Design review of the part built by this model. Coordinates are the model's own, in mm. A direction names the side the tool comes from. Coordinates: 2 decimals unless noted, no trailing zeros. Write each loop counter-clockwise with the first axis right and the second up, starting at its lowest first coordinate (ties: lowest second). Pieces come first, ordered by that corner, then holes.
Q1. Clearance check with flat-ended pins moving along their axes: pin 1 Ø1.5 at (x, y) = (-10, 11.5) entering from -Z; pin 2 Ø11 at (x, z) = (-7.5, 50) entering from +Y; pin 3 Ø8 at (x, z) = (-38, -37) entering from +Y (3 decimals); pin 4 Ø2 at (x, z) = (-34.925, 34.925) entering from -Y. State where each tip first meets the part, or that it passes through.
Q2. Add section B-B, the plane y = 13. Give the boundary of the cut face in (x, z) (3 decimals), plus the area to 3 significant figures.
Q3. Machinability: for faces 1 (the face through (-41, 6.35, -41)), 2 (the face through (47.625, 3, -32)), 3 (the face through (35.274, 4.994, -42.855)), which of the approach directions +Z, -Z, +X, -X, +Y, -Y give a long, thin tool a straight path to every point of the face, cutting with its end or side? Answer none if there is none.
Q4. To check wall thickness, follow probe 1 along Z at (x, y) = (-25, 6.75); probe 2 along X at (y, z) = (7.75, 26); probe 3 along Y at (x, z) = (-9, 43). State the ranges of each line that lie inside material, in increasing order.
from build123d import *

# Parameters (mm, degrees)
SKETCH1_W               = 95.25
SKETCH1_H               = 95.25
SKETCH1_R               = 37.465
BOSS_EXTRUDE1_DEPTH     = 6.35
SKETCH2_R               = 1.75
CUT_EXTRUDE1_DEPTH      = 68.650600515
CIRPATTERN1_COUNT       = 4
FILLET1_R               = 12.7
FILLET2_R               = 3.175
SKETCH5_R               = 55.5625
SKETCH5_R_2             = 44.45
SKETCH5_R_3             = 1.75
BOSS_EXTRUDE2_DEPTH     = 6.35
BOSS_EXTRUDE4_START     = 1.5875
SKETCH8_R               = 55.5625
SKETCH8_R_2             = 52.3875
BOSS_EXTRUDE4_DEPTH     = 1.5875
CUT_EXTRUDE3_DEPTH      = 80.152437976
CUT_EXTRUDE3_DEPTH_BACK = 3.175
SKETCH10_R              = 7.9375


with BuildPart() as part:
    # Sketch1 → Boss-Extrude1 (new body)
    with BuildSketch(Plane(origin=(0, 0, 0), x_dir=(1, 0, 0), z_dir=(0, 1, 0))):
        Rectangle(SKETCH1_W, SKETCH1_H)
        with Locations(Location((0, 0, 0), (0, 0, 270))):
            Circle(SKETCH1_R, mode=Mode.SUBTRACT)
    extrude(amount=BOSS_EXTRUDE1_DEPTH)

    # Sketch2 → Cut-Extrude1 (cut, through all)
    with BuildSketch(Plane(origin=(0, 6.35, 0), x_dir=(1, 0, 0), z_dir=(0, 1, 0))):
        with Locations(Location((-34.925, 34.925, 0), (0, 0, 270))):
            Circle(SKETCH2_R)
    cut_extrude1 = extrude(amount=-CUT_EXTRUDE1_DEPTH, mode=Mode.SUBTRACT)

    # CirPattern1: Cut-Extrude1 ×4 about axis
    cirpattern1_axis = Axis((0, 0, 0), (0, 1, 0))
    for i in range(1, CIRPATTERN1_COUNT):
        add(cut_extrude1.rotate(cirpattern1_axis, i * 360 / CIRPATTERN1_COUNT), mode=Mode.SUBTRACT)

    # Fillet1
    fillet1_edges = [part.edges().sort_by_distance(p)[0] for p in [
        (-47.625, 3.175, -47.625),
        (47.625, 3.175, -47.625),
        (47.625, 3.175, 47.625),
        (-47.625, 3.175, 47.625),
    ]]
    fillet(fillet1_edges, radius=FILLET1_R)

    # Sketch4 → Revolve1 (revolve)
    with BuildSketch(Plane.XY, mode=Mode.PRIVATE) as revolve1_sk:
        Polygon((37.465, 12.7), (37.465, 6.35), (38.1, 6.35), (38.1, 10.3505), (38.1, 14.2875), (37.465, 15.875), align=None)
    revolve(revolve1_sk.sketch.rotate(Axis((0, 0, 0), (0, 1, 0)), 90), axis=Axis((0, 0, 0), (0, 1, 0)))

    # Fillet2
    fillet2_edges = [part.edges().sort_by_distance(p)[0] for p in [
        (0, 6.35, 38.1),
    ]]
    fillet(fillet2_edges, radius=FILLET2_R)

    # Sketch5 → Boss-Extrude2 (add, through all)
    with BuildSketch(Plane(origin=(0, 6.35, 0), x_dir=(1, 0, 0), z_dir=(0, 1, 0))):
        Circle(SKETCH5_R)
        Circle(SKETCH5_R_2, mode=Mode.SUBTRACT)
        with Locations(Location((-34.925, 34.925, 0), (0, 0, 270))):
            Circle(SKETCH5_R_3, mode=Mode.SUBTRACT)
        with Locations((-34.925, -34.925)):
            Circle(SKETCH5_R_3, mode=Mode.SUBTRACT)
        with Locations(Location((34.925, -34.925, 0), (0, 0, 90))):
            Circle(SKETCH5_R_3, mode=Mode.SUBTRACT)
        with Locations(Location((34.925, 34.925, 0), (0, 0, 180))):
            Circle(SKETCH5_R_3, mode=Mode.SUBTRACT)
    extrude(amount=-BOSS_EXTRUDE2_DEPTH)

    # Sketch8 → Boss-Extrude4 (add)
    with BuildSketch(Plane(origin=(0, 6.35, 0), x_dir=(1, 0, 0), z_dir=(0, 1, 0)).offset(BOSS_EXTRUDE4_START)):
        with Locations(Location((0, 0, 0), (0, 0, 270))):
            Circle(SKETCH8_R)
        with Locations(Location((0, 0, 0), (0, 0, 270))):
            Circle(SKETCH8_R_2, mode=Mode.SUBTRACT)
    extrude(amount=-BOSS_EXTRUDE4_DEPTH)

    # Sketch10 → Cut-Extrude3 (cut, two sides: drawn at the far end of the back side and taken through both)
    with BuildSketch(Plane(origin=(0, 6.35, 0), x_dir=(1, 0, 0), z_dir=(0, 1, 0)).offset(-CUT_EXTRUDE3_DEPTH_BACK)):
        with Locations(Location((-34.925, 34.925, 0), (0, 0, 270))):
            Circle(SKETCH10_R)
        with Locations(Location((34.925, 34.925, 0), (0, 0, 270))):
            Circle(SKETCH10_R)
        with Locations(Location((34.925, -34.925, 0), (0, 0, 270))):
            Circle(SKETCH10_R)
        with Locations(Location((-34.925, -34.925, 0), (0, 0, 270))):
            Circle(SKETCH10_R)
    extrude(amount=CUT_EXTRUDE3_DEPTH + CUT_EXTRUDE3_DEPTH_BACK, mode=Mode.SUBTRACT)


solid = part.part
Here are the results:
1. pin 1: stops at z = -36.96
1. pin 2: stops at y = 7.94
1. pin 3: stops at y = 3.175
1. pin 4: passes through
2. outline: circle Ø76.2 at (0, 0); hole circle Ø74.93 at (0, 0)
2. area: 151 mm2
3. face 1: -Z, -X, +Y
3. face 2: -Z, +X, +Y, -Y
3. face 3: +Y
4. probe 1: z = -49.62 to -46.04, -30.88 to -27.9, 27.9 to 30.88, 46.04 to 49.62
4. probe 2: x = -49.1 to -45.48, -28.59 to -26.97, 26.97 to 28.59, 45.48 to 49.1
4. probe 3: y = 0 to 6.35
